from build123d import *

# Parameters (mm, degrees)
BOSS_EXTRUDE2_DEPTH      = 8
SKETCH2_W                = 81
SKETCH2_H                = 89.6
BOSS_EXTRUDE3_DEPTH      = 2
SKETCH3_R                = 1.75
CUT_EXTRUDE1_DEPTH       = 125.5538661
CUT_EXTRUDE2_DEPTH       = 124.262587838
CUT_EXTRUDE2_DEPTH_BACK  = 124.262587838
SKETCH4_W                = 80.6
SKETCH4_H                = 6.1
SKETCH5_W                = 68.8
SKETCH5_H                = 1.2
BOSS_EXTRUDE4_DEPTH      = 2
FILLET2_R                = 2
BOSS_EXTRUDE5_DEPTH      = 1.5
BOSS_EXTRUDE5_DEPTH_BACK = 1.5
SKETCH7_R                = 1.25
FILLET5_R                = 1


with BuildPart() as part:
    # Sketch1 → Boss-Extrude2 (new body)
    with BuildSketch(Plane(origin=(0, 0, 0), x_dir=(1, 0, 0), z_dir=(0, 1, 0))):
        Polygon((-46.14154214, 4.488604838), (-46.14154214, 13.488604838), (-46.14154214, 92.088604838), (30.85845786, 92.088604838), (30.85845786, 13.488604838), (30.85845786, 4.488604838), (32.85845786, 4.488604838), (32.85845786, 94.088604838), (-48.14154214, 94.088604838), (-48.14154214, 4.488604838), align=None)
    extrude(amount=BOSS_EXTRUDE2_DEPTH)

    # Sketch2 → Boss-Extrude3 (add)
    with BuildSketch(Plane(origin=(0, 8, 0), x_dir=(1, 0, 0), z_dir=(0, 1, 0))):
        with Locations((-7.64154214, 49.288604838)):
            Rectangle(SKETCH2_W, SKETCH2_H)
    extrude(amount=BOSS_EXTRUDE3_DEPTH)

    # Sketch3 → Cut-Extrude1 (cut, through all)
    with BuildSketch(Plane(origin=(32.85845786, 0, 0), x_dir=(0, 0, -1), z_dir=(1, 0, 0))):
        with Locations((9.238604838, 3.6)):
            Circle(SKETCH3_R)
    extrude(amount=-CUT_EXTRUDE1_DEPTH, mode=Mode.SUBTRACT)

    # Sketch4 → Cut-Extrude2 (cut, two sides: drawn at the far end of the back side and taken through both)
    with BuildSketch(Plane.ZY.offset(-30.85845786).offset(-CUT_EXTRUDE2_DEPTH_BACK)):
        with Locations((-53.788604838, 3.05)):
            Rectangle(SKETCH4_W, SKETCH4_H)
    extrude(amount=CUT_EXTRUDE2_DEPTH + CUT_EXTRUDE2_DEPTH_BACK, mode=Mode.SUBTRACT)

    # Sketch5 → Boss-Extrude4 (add)
    with BuildSketch(Plane.XZ.offset(-8)):
        with Locations((-7.64154214, -12.405302831)):
            Rectangle(SKETCH5_W, SKETCH5_H)
    extrude(amount=BOSS_EXTRUDE4_DEPTH)

    # Fillet2
    fillet2_edges = [part.edges().sort_by_distance(p)[0] for p in [
        (-7.64154214, 8, -11.805302831),
        (-47.14154214, 0, -4.488604838),
        (-47.14154214, 0, -13.488604838),
        (-47.14154214, 6.1, -13.488604838),
        (31.85845786, 6.1, -13.488604838),
        (31.85845786, 0, -4.488604838),
        (31.85845786, 0, -13.488604838),
    ]]
    fillet(fillet2_edges, radius=FILLET2_R - 0.0001)  # a hair under: the kernel refuses the full size

    # Sketch7 → Boss-Extrude5 (add, two sides: drawn at the far end of the back side and taken through both)
    with BuildSketch(Plane.ZY.offset(7.64154214).offset(-BOSS_EXTRUDE5_DEPTH_BACK)):
        with BuildLine():
            Line((-94.088604838, 10), (-98.088604838, 10))
            ThreePointArc((-98.088604838, 10), (-98.79571162, 9.707106781), (-99.088604838, 9))
            Line((-99.088604838, 9), (-99.088604838, 7.1))
            ThreePointArc((-99.088604838, 7.1), (-98.79571162, 6.392893219), (-98.088604838, 6.1))
            Line((-98.088604838, 6.1), (-94.088604838, 6.1))
            Line((-94.088604838, 6.1), (-94.088604838, 10))
        make_face()
        with Locations((-96.588604838, 8.05)):
            Circle(SKETCH7_R, mode=Mode.SUBTRACT)
    extrude(amount=BOSS_EXTRUDE5_DEPTH + BOSS_EXTRUDE5_DEPTH_BACK)

    # Fillet5
    fillet5_edges = [part.edges().sort_by_distance(p)[0] for p in [
        (-6.14154214, 8.05, -94.088604838),
        (-9.14154214, 8.05, -94.088604838),
    ]]
    fillet(fillet5_edges, radius=FILLET5_R)


solid = part.part
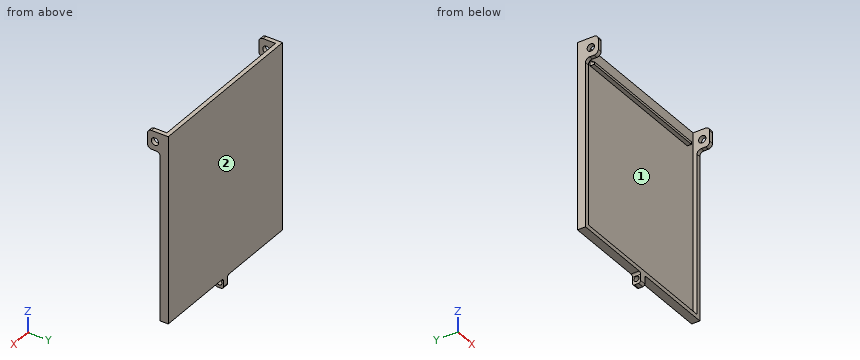
Geometry: final body of the model. Coordinates: model frame, mm. Face numbers are marked on the shaded views. Give positions to 0.01 mm unless a question says otherwise; leave off trailing zeros. Write each loop counter-clockwise with the first axis right and the second up, starting at its lowest first coordinate (ties: lowest second). Pieces come first, ordered by that corner, then holes. Notation, with made-up numbers: (76.5, -19) - (113.5, -19) arc R14 cw to (113.5, -6) - close; hole circle Ø2 at (-38, 59.25). An arc over 180 degrees is marked (long way). Return JSON: item names as keys, results as strings. Group by question number.
1) Mould query, pull axis X, two halves, no side actions, for the marked faces 1 and 2. Classes: released by +X, released by -X, zero draft, split by the parting line, or undercut.
2) Line query: line 1 (X direction, y = 5.25, z = -12); line 2 (Y direction, x = 16, z = -26); line 3 (Y direction, x = 4, z = -92.5). Output: solid intervals per line, ascending.
3) First-contact query: P1, Ø2, axis at x = -4.5, z = -22, coming from the -Y side; P2, Ø4.5, axis at y = 8.5, z = -97.5, coming from the +X side; P3, Ø2, axis at x = 13, y = 8, coming from the -Z side. Flat tips, straight axial feed; report the tip coordinate or a pass-through.
4) Section B-B on z = -24. Return the cut outline in (x, y), plus the area to 3 significant figures.
Filled in:
{
 "1": {"face 1": "undercut", "face 2": "zero draft"},
 "2": {"line 1": "x = -48.14 to -46.14, 30.86 to 32.86", "line 2": "y = 8 to 10", "line 3": "y = 6.1 to 10"},
 "3": {"P1": "stops at y = 8", "P2": "stops at x = -6.14", "P3": "stops at z = -94.09"},
 "4": {"outline": "(-48.14, 6.1) - (-46.14, 6.1) - (-46.14, 8) - (30.86, 8) - (30.86, 6.1) - (32.86, 6.1) - (32.86, 10) - (-48.14, 10) - close", "area": "170 mm^2"}
}
